Geometry check sheet. Reference: the model listing, model coordinates, mm. Face numbers are marked on the shaded views. A direction names the side the tool comes from. Coordinates: 2 decimals unless noted, no trailing zeros. Loops run counter-clockwise (first coordinate to the right, second up) from the corner with the lowest first, then second, coordinate; pieces in that order, holes last. Notation, with made-up numbers: (6, 5) - (10, 5) arc R6 cw to (10, 16) - close; hole circle Ø2 at (15.25, 7.5). An arc over 180 degrees is marked (long way). One line per item, written item: value.
from build123d import *

# Parameters (mm, degrees)
SCHIZZO1_W                    = 85.2
SCHIZZO1_H                    = 85.6
SCHIZZO1_R                    = 2
ESTRUSIONE_ESTRUSIONE1_DEPTH  = 1.6
SCHIZZO3_W                    = 15.2
SCHIZZO3_H                    = 9
ESTRUSIONE_ESTRUSIONE2_DEPTH  = 5.6
SCHIZZO4_W                    = 14
SCHIZZO4_H                    = 13
ESTRUSIONE_ESTRUSIONE3_DEPTH  = 12
SCHIZZO5_W                    = 9.6
SCHIZZO5_H                    = 12
ESTRUSIONE_ESTRUSIONE4_DEPTH  = 5.5
SCHIZZO6_R                    = 2.5
SCHIZZO6_R_2                  = 1.5
ESTRUSIONE_SOTTILE1_DEPTH     = 3
SCHIZZO7_W                    = 16
SCHIZZO7_H                    = 14.5
ESTRUSIONE_ESTRUSIONE5_DEPTH  = 2.5
SCHIZZO8_W                    = 8.7
SCHIZZO8_H                    = 7.8
ESTRUSIONE_ESTRUSIONE6_DEPTH  = 3.8
SCHIZZO9_W                    = 14.2
SCHIZZO9_H                    = 9.2
ESTRUSIONE_ESTRUSIONE7_DEPTH  = 11
SCHIZZO10_R                   = 3.2
TAGLIO_ESTRUSIONE1_DEPTH      = 10
SCHIZZO11_W                   = 4.4
SCHIZZO11_H                   = 31
ESTRUSIONE_ESTRUSIONE8_DEPTH  = 11
ESTRUSIONE_ESTRUSIONE9_DEPTH  = 5.5
SCHIZZO14_R                   = 1.5
TAGLIO_ESTRUSIONE2_DEPTH      = 5.5
SCHIZZO15_W                   = 16.4
SCHIZZO15_H                   = 26
ESTRUSIONE_ESTRUSIONE10_DEPTH = 14
SCHIZZO16_W                   = 13.3
SCHIZZO16_H                   = 16.5
ESTRUSIONE_ESTRUSIONE11_DEPTH = 15.5
SCHIZZO17_W                   = 7.3
SCHIZZO17_H                   = 13
SCHIZZO17_W_2                 = 5
SCHIZZO17_H_2                 = 35.6
ESTRUSIONE_ESTRUSIONE12_DEPTH = 3.9


with BuildPart() as part:
    # Schizzo1 → Estrusione-Estrusione1 (new body)
    with BuildSketch(Plane.XY):
        Rectangle(SCHIZZO1_W, SCHIZZO1_H)
        with Locations((-38.8, 36)):
            Circle(SCHIZZO1_R, mode=Mode.SUBTRACT)
        with Locations((32.6, 36)):
            Circle(SCHIZZO1_R, mode=Mode.SUBTRACT)
        with Locations((-38.8, -32.8)):
            Circle(SCHIZZO1_R, mode=Mode.SUBTRACT)
        with Locations((32.6, -32.8)):
            Circle(SCHIZZO1_R, mode=Mode.SUBTRACT)
    extrude(amount=ESTRUSIONE_ESTRUSIONE1_DEPTH)

    # Schizzo3 → Estrusione-Estrusione2 (add)
    with BuildSketch(Plane.XY.offset(1.6)):
        with Locations((-26.4, 39.3)):
            Rectangle(SCHIZZO3_W, SCHIZZO3_H)
    extrude(amount=ESTRUSIONE_ESTRUSIONE2_DEPTH)

    # Schizzo4 → Estrusione-Estrusione3 (add)
    with BuildSketch(Plane.XY.offset(1.6)):
        with Locations((-5.6, 36.3)):
            Rectangle(SCHIZZO4_W, SCHIZZO4_H)
    extrude(amount=ESTRUSIONE_ESTRUSIONE3_DEPTH)

    # Schizzo5 → Estrusione-Estrusione4 (add)
    with BuildSketch(Plane.XY.offset(1.6)):
        with Locations((8.2, 36.8)):
            Rectangle(SCHIZZO5_W, SCHIZZO5_H)
        with Locations((22.2, 36.8)):
            Rectangle(SCHIZZO5_W, SCHIZZO5_H)
    extrude(amount=ESTRUSIONE_ESTRUSIONE4_DEPTH)

    # Schizzo6 → Estrusione-Sottile1 (add)
    # profile 1 of 2: a face of its own
    with BuildSketch(Plane(origin=(0, 42.8, 0), x_dir=(1, 0, 0), z_dir=(0, 1, 0))):
        with Locations((8.2, -4.35)):
            Circle(SCHIZZO6_R)
        with Locations((8.2, -4.35)):
            Circle(SCHIZZO6_R_2, mode=Mode.SUBTRACT)
    # profile 2 of 2: a face of its own
    with BuildSketch(Plane(origin=(0, 42.8, 0), x_dir=(1, 0, 0), z_dir=(0, 1, 0))):
        with Locations((22.2, -4.35)):
            Circle(SCHIZZO6_R)
        with Locations((22.2, -4.35)):
            Circle(SCHIZZO6_R_2, mode=Mode.SUBTRACT)
    extrude(amount=ESTRUSIONE_SOTTILE1_DEPTH)

    # Schizzo7 → Estrusione-Estrusione5 (add)
    with BuildSketch(Plane(origin=(0, 0, 0), x_dir=(-1, 0, 0), z_dir=(0, 0, -1))):
        with Locations((-34.6, 23.75)):
            Rectangle(SCHIZZO7_W, SCHIZZO7_H)
    extrude(amount=ESTRUSIONE_ESTRUSIONE5_DEPTH)

    # Schizzo8 → Estrusione-Estrusione6 (add)
    with BuildSketch(Plane.XY.offset(1.6)):
        with Locations((39.25, 10.4)):
            Rectangle(SCHIZZO8_W, SCHIZZO8_H)
    extrude(amount=ESTRUSIONE_ESTRUSIONE6_DEPTH)

    # Schizzo9 → Estrusione-Estrusione7 (add)
    with BuildSketch(Plane.XY.offset(1.6)):
        with Locations((37.5, -1.8)):
            Rectangle(SCHIZZO9_W, SCHIZZO9_H)
    extrude(amount=ESTRUSIONE_ESTRUSIONE7_DEPTH)

    # Schizzo10 → Taglio-Estrusione1 (cut)
    with BuildSketch(Plane(origin=(44.6, 0, 0), x_dir=(0, 0, -1), z_dir=(1, 0, 0))):
        with Locations((-8.163212145, -1.8)):
            Circle(SCHIZZO10_R)
    extrude(amount=-TAGLIO_ESTRUSIONE1_DEPTH, mode=Mode.SUBTRACT)

    # Schizzo11 → Estrusione-Estrusione8 (add)
    with BuildSketch(Plane.XY.offset(1.6)):
        with Locations((40.4, -27.3)):
            Rectangle(SCHIZZO11_W, SCHIZZO11_H)
    extrude(amount=ESTRUSIONE_ESTRUSIONE8_DEPTH)

    # Schizzo12 → Estrusione-Estrusione9 (add)
    with BuildSketch(Plane(origin=(42.6, 0, 0), x_dir=(0, 0, -1), z_dir=(1, 0, 0))):
        with BuildLine():
            Line((-11.1, -34.225), (-11.1, -20.375))
            ThreePointArc((-11.1, -20.375), (-10.537042571, -19.203696786), (-9.270731707, -18.911585366))
            Line((-9.270731707, -18.911585366), (-4.270731707, -20.036585366))
            ThreePointArc((-4.270731707, -20.036585366), (-3.428696786, -20.562957429), (-3.1, -21.5))
            Line((-3.1, -21.5), (-3.1, -33.1))
            ThreePointArc((-3.1, -33.1), (-3.428696786, -34.037042571), (-4.270731707, -34.563414634))
            Line((-4.270731707, -34.563414634), (-9.270731707, -35.688414634))
            ThreePointArc((-9.270731707, -35.688414634), (-10.537042571, -35.396303214), (-11.1, -34.225))
        make_face()
    extrude(amount=ESTRUSIONE_ESTRUSIONE9_DEPTH)

    # Schizzo14 → Taglio-Estrusione2 (cut)
    with BuildSketch(Plane(origin=(42.6, 0, 0), x_dir=(0, 0, -1), z_dir=(1, 0, 0))):
        with Locations((-7.1, -14.8)):
            Circle(SCHIZZO14_R)
        with Locations((-7.1, -39.8)):
            Circle(SCHIZZO14_R)
    extrude(amount=-TAGLIO_ESTRUSIONE2_DEPTH, mode=Mode.SUBTRACT)

    # Schizzo15 → Estrusione-Estrusione10 (add)
    with BuildSketch(Plane.XY.offset(1.6)):
        with Locations((19.6, -34.1)):
            Rectangle(SCHIZZO15_W, SCHIZZO15_H)
    extrude(amount=ESTRUSIONE_ESTRUSIONE10_DEPTH)

    # Schizzo16 → Estrusione-Estrusione11 (add)
    with BuildSketch(Plane.XY.offset(1.6)):
        with Locations((-27.05, -38.15)):
            Rectangle(SCHIZZO16_W, SCHIZZO16_H)
        with Locations((-4.75, -38.15)):
            Rectangle(SCHIZZO16_W, SCHIZZO16_H)
    extrude(amount=ESTRUSIONE_ESTRUSIONE11_DEPTH)

    # Schizzo17 → Estrusione-Estrusione12 (add)
    with BuildSketch(Plane(origin=(0, 0, 0), x_dir=(-1, 0, 0), z_dir=(0, 0, -1))):
        with Locations((36.55, 18)):
            Rectangle(SCHIZZO17_W, SCHIZZO17_H)
        with Locations((36.9, -9)):
            Rectangle(SCHIZZO17_W_2, SCHIZZO17_H_2)
    extrude(amount=ESTRUSIONE_ESTRUSIONE12_DEPTH)


solid = part.part
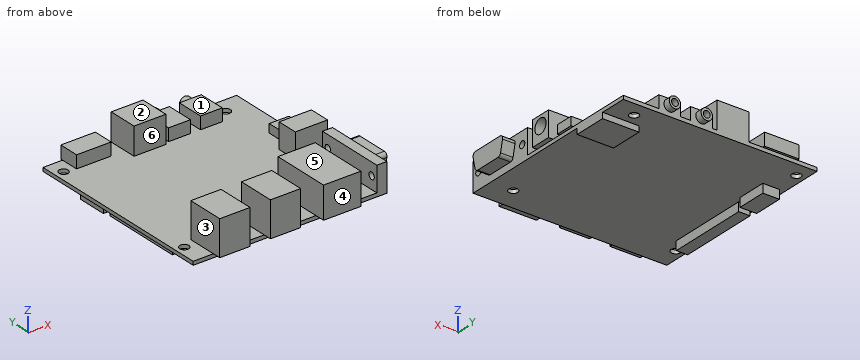
(1) Cross-section at C-C on y = -17.5. Record the cut outline in (x, z).
Reply:
outline: (-42.6, 0) - (-39.4, 0) - (-39.4, -3.9) - (-34.4, -3.9) - (-34.4, 0) - (42.6, 0) - (42.6, 12.6) - (38.2, 12.6) - (38.2, 1.6) - (-42.6, 1.6) - close
(2) Material ranges on probe 1 along Y at (x, z) = (32.6, 0.7); probe 2 along X at (y, z) = (45.1, 4.35); probe 3 along X at (y, z) = (43.75, 4.35), recorded low to high. Write a range as from..to.
Reply:
probe 1: -42.8..-34.8, -30.8..34, 38..42.8
probe 2: 5.7..6.7, 9.7..10.7, 19.7..20.7, 23.7..24.7
probe 3: -34..-18.8, 5.7..6.7, 9.7..10.7, 19.7..20.7, 23.7..24.7
(3) Cross-section at A-A on x = 32.6. Record the cut outline in (y, z), and give its area (3 significant figures).
Reply:
outline: (-42.8, 0) - (-34.8, 0) - (-34.8, 1.6) - (-42.8, 1.6) - close; (-30.8, 0) - (16.5, 0) - (16.5, -2.5) - (31, -2.5) - (31, 0) - (34, 0) - (34, 1.6) - (2.8, 1.6) - (2.8, 12.6) - (-6.4, 12.6) - (-6.4, 1.6) - (-30.8, 1.6) - close; (38, 0) - (42.8, 0) - (42.8, 1.6) - (38, 1.6) - close
area: 262 mm2
(4) Release check for a two-part mould opening along Y. For the marked faces 4, 5 and 6 record: pulls with the +Y half, pulls with the -Y half, needs draft (parallel to the pull), parting line crosses it, or undercut.
Reply:
face 4: pulls with the -Y half
face 5: needs draft
face 6: undercut
(5) Cross-section at B-B on y = -39.8. Record the cut outline in (x, z).
Reply:
outline: (-42.6, 0) - (42.6, 0) - (42.6, 5.6) - (38.2, 5.6) - (38.2, 1.6) - (27.8, 1.6) - (27.8, 15.6) - (11.4, 15.6) - (11.4, 1.6) - (1.9, 1.6) - (1.9, 17.1) - (-11.4, 17.1) - (-11.4, 1.6) - (-20.4, 1.6) - (-20.4, 17.1) - (-33.7, 17.1) - (-33.7, 1.6) - (-42.6, 1.6) - close; (38.2, 8.6) - (42.6, 8.6) - (42.6, 12.6) - (38.2, 12.6) - close
(6) Go/stop test with flat-tipped pins: pin 1 Ø6 at (x, z) = (-9, 8.5) entering from -Y; pin 2 Ø2 at (x, z) = (40, 9) entering from +Y; pin 3 Ø3.5 at (y, z) = (-28, 6) entering from -X; pin 4 Ø3 at (x, y) = (-38.8, 36) entering from +Z. Record where each tip stops, or that it passes through.
Reply:
pin 1: y = -46.4
pin 2: y = 2.8
pin 3: x = 11.4
pin 4: through
(7) Access from +Z, -Z, +X, -X, +Y, -Y to the whole of each face (thin tool, end or side, straight path). Record for the marked faces 1, 2 and 3.
Reply:
face 1: +Z, +X, +Y
face 2: +Z, +X, -X, +Y
face 3: +Z, -X, -Y
(8) Cross-section at D-D on x = -23.5. Record the cut outline in (y, z), and give its area (3 significant figures).
Reply:
outline: (-46.4, 1.6) - (-42.8, 1.6) - (-42.8, 0) - (42.8, 0) - (42.8, 1.6) - (43.8, 1.6) - (43.8, 7.2) - (34.8, 7.2) - (34.8, 1.6) - (-29.9, 1.6) - (-29.9, 17.1) - (-46.4, 17.1) - close
area: 443 mm2
